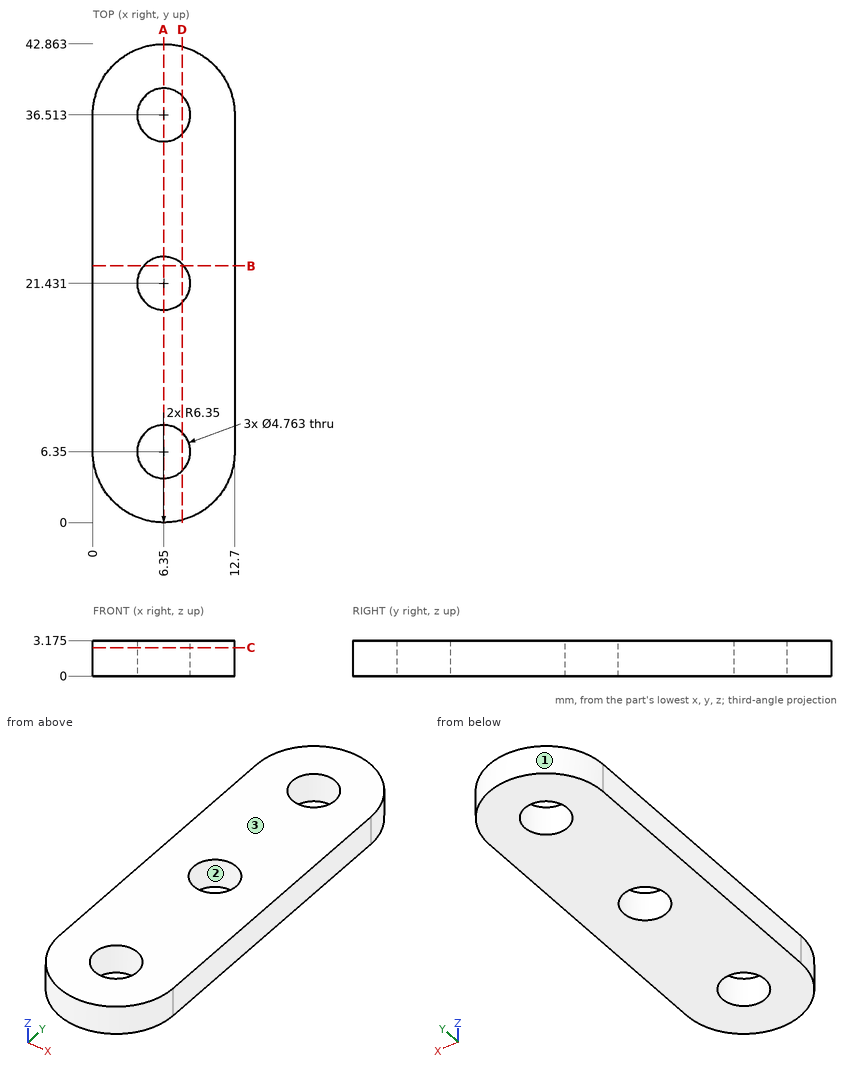
Design review of the part shown in the three views and the two pictorial views. Dimensions are in mm from the part's minimum x, y and z. Round coordinates to 2 decimals unless told otherwise and drop trailing zeros. Order: outer loops, then holes, each group sorted by start corner. A loop starts at its lowest first (then second) coordinate and runs counter-clockwise, first axis right, second up.
Item 1: For pin 1 (5 mm diameter, centred on x = 6, y = 23, fed in from +Z) (1 decimal); pin 2 (3 mm diameter, centred on x = 6.35, y = 6.35, fed in from +Z), all flat-tipped, find the tip position at first contact; note any pin that passes through.
Working result:
pin 1: stops at z = 3.2
pin 2: passes through
Item 2: To check wall thickness, follow probe 1 along Y at (x, z) = (6.35, 1.5); probe 2 along X at (y, z) = (36.5, 0.85); probe 3 along Y at (x, z) = (5.75, 1) (1 decimal). State the ranges of each line that lie inside material, in increasing order.
Working result:
probe 1: y = 0 to 3.97, 8.73 to 19.05, 23.81 to 34.13, 38.89 to 42.86
probe 2: x = 0 to 3.97, 8.73 to 12.7
probe 3: y = 0 to 4, 8.7 to 19.1, 23.7 to 34.2, 38.8 to 42.8
Item 3: Draft analysis for pull direction Y (two halves, no side actions). For the marked faces 1, 2 and 3, state which applies: released by +Y, released by -Y, zero draft, split by the parting line, or undercut.
Working result:
face 1: released by +Y
face 2: undercut
face 3: zero draft
Item 4: Add section D-D, the plane x = 8. State the section outline as (y, z) points (1 decimal).
Working result:
outline: (0.2, 0) - (4.6, 0) - (4.6, 3.2) - (0.2, 3.2) - close; (8.1, 0) - (19.7, 0) - (19.7, 3.2) - (8.1, 3.2) - close; (23.1, 0) - (34.8, 0) - (34.8, 3.2) - (23.1, 3.2) - close; (38.2, 0) - (42.6, 0) - (42.6, 3.2) - (38.2, 3.2) - close
Item 5: Add section A-A, the plane x = 6.35. Count the separate pieces of the cut face and the enclosed holes in it.
Working result:
separate pieces: 4
enclosed holes: 0
Item 6: Add section B-B, the plane y = 23. State the section outline as (x, z) points (1 decimal).
Working result:
outline: (0, 0) - (4.6, 0) - (4.6, 3.2) - (0, 3.2) - close; (8.1, 0) - (12.7, 0) - (12.7, 3.2) - (8.1, 3.2) - close
Item 7: Add section C-C, the plane z = 2.55. State the section outline as (x, y) points, and give its area (3 significant figures).
Working result:
outline: (0, 6.35) arc R6.35 ccw to (12.7, 6.35) - (12.7, 36.51) arc R6.35 ccw to (0, 36.51) - close; hole circle Ø4.76 at (6.35, 6.35); hole circle Ø4.76 at (6.35, 21.43); hole circle Ø4.76 at (6.35, 36.51)
area: 456 mm2
